from build123d import *

# Parameters (mm, degrees)
SKETCH1_R           = 17
SKETCH2_R           = 6.5
SKETCH3_R           = 6.5
SKETCH3_R_2         = 5
BOSS_EXTRUDE1_DEPTH = 80
SHELL1_T            = -3
SKETCH4_R           = 5.3
CUT_EXTRUDE1_DEPTH  = 80
SKETCH5_R           = 17
SKETCH5_R_2         = 12.65
BOSS_EXTRUDE2_DEPTH = 15


with BuildPart() as part:
    # Sketch1 → Loft1 section 0
    with BuildSketch(Plane.XY):
        Circle(SKETCH1_R)
    # Sketch2 → Loft1 section 1
    with BuildSketch(Plane.XY.offset(10)):
        Circle(SKETCH2_R)
    loft()

    # Sketch3 → Boss-Extrude1 (add)
    with BuildSketch(Plane.XY.offset(10)):
        Circle(SKETCH3_R)
        Circle(SKETCH3_R_2, mode=Mode.SUBTRACT)
    extrude(amount=BOSS_EXTRUDE1_DEPTH)

    # Shell1
    shell1_openings = [part.faces().sort_by_distance(p)[0] for p in [
        (0, 0, 0),
    ]]
    offset(amount=SHELL1_T, openings=shell1_openings, kind=Kind.INTERSECTION)

    # Sketch4 → Cut-Extrude1 (cut)
    with BuildSketch(Plane(origin=(0, 0, 7), x_dir=(-1, 0, 0), z_dir=(0, 0, -1))):
        Circle(SKETCH4_R)
    extrude(amount=-CUT_EXTRUDE1_DEPTH, mode=Mode.SUBTRACT)

    # Sketch5 → Boss-Extrude2 (add)
    with BuildSketch(Plane(origin=(0, 0, 0), x_dir=(-1, 0, 0), z_dir=(0, 0, -1))):
        Circle(SKETCH5_R)
        Circle(SKETCH5_R_2, mode=Mode.SUBTRACT)
    extrude(amount=BOSS_EXTRUDE2_DEPTH)


solid = part.part
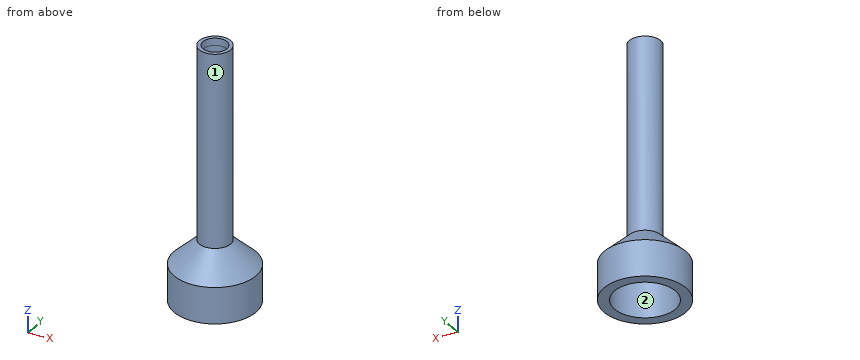
Here's how the part is built. I have some questions about the finished solid (model axes, mm). Face numbers are marked on the shaded views. Round coordinates to 2 decimals unless told otherwise and drop trailing zeros. Loops run counter-clockwise (first coordinate to the right, second up) from the corner with the lowest first, then second, coordinate; pieces in that order, holes last.
1. We'd pull the mould along Y, two halves only. Please class the marked faces 1 and 2: +Y half, -Y half, draft (parallel to the pull), parting line (faces both ways), or undercut.
Answer list:
face 1: parting line
face 2: undercut
2. If we section it at B-B on z = 12: Write out the boundary of the cut face in (x, y), plus the area to 3 significant figures.
Answer list:
outline: circle Ø13 at (0, 0); hole circle Ø10.6 at (0, 0)
area: 44.5 mm2
3. If we section it at A-A on x = 0: Write out the boundary of the cut face in (y, z), plus the area to 3 significant figures.
Answer list:
outline: (-17, -15) - (-12.65, -15) - (-12.65, 0) - (-5.3, 7) - (-5.3, 87) - (-5, 87) - (-5, 90) - (-6.5, 90) - (-6.5, 10) - (-17, 0) - close; (5, 87) - (5.3, 87) - (5.3, 7) - (12.65, 0) - (12.65, -15) - (17, -15) - (17, 0) - (6.5, 10) - (6.5, 90) - (5, 90) - close
area: 402 mm2
4. For P1, Ø10, axis at y = -7, z = 1, coming from the -X side; P2, Ø8.5, axis at x = -1.5, y = -1, coming from the -Z side; P3, Ø1.5, axis at x = -10, y = 4.5, coming from the -Z side, each with a flat end and sliding along its axis, tell me the tip position at first contact or that it passes through.
Answer list:
P1: stops at x = -16.87
P2: stops at z = 6.28
P3: stops at z = 0.89
5. If we section it at C-C on z = -2.5: Write out the boundary of the cut face in (x, y).
Answer list:
outline: circle Ø34 at (0, 0); hole circle Ø25.3 at (0, 0)
6. If I drill on line 1 along X through (y, z) = (0, -8); line 2 along Y through (x, z) = (0, 87.7), over which ranges is the centre line in solid material (lowest first)?
Answer list:
line 1: x = -17 to -12.65, 12.65 to 17
line 2: y = -6.5 to -5, 5 to 6.5
